Work out the finished part from the listing and answer in its coordinate system (mm). Face numbers are marked on the shaded views. A direction names the side the tool comes from. Coordinates: 2 decimals unless noted, no trailing zeros. Order: outer loops, then holes, each group sorted by start corner. A loop starts at its lowest first (then second) coordinate and runs counter-clockwise, first axis right, second up. Notation, with made-up numbers: M 60,23.25 L 75,23.25 A17 cw 75,35.25 Z; hole C -22.5,34 d4. An arc over 180 degrees is marked long. Answer in a Markdown table with one row per item. Add a question column.
Item 1: The part is cut by section A-A (x = 0). Write down the section's boundary in (y, z).
Item 2: Which of the six approach directions +Z, -Z, +X, -X, +Y, -Y give full straight-line access (tool end or side, diameter ignored) to the marked faces 1 and 2?
Item 3: The part is cut by section C-C (y = 11). Write down the section's boundary in (x, z), then the cut area to 3 significant figures.
Item 4: Flat-ended cylindrical pins translate along their axes: pin 1 Ø12 at (x, y) = (27.5, 4) entering from -Z; pin 2 Ø8 at (x, z) = (5.79, -4.21) entering from +Y; pin 3 Ø4 at (x, y) = (27, 4.5) entering from +Z; pin 4 Ø13.5 at (x, z) = (0, 0) entering from +Y. Find the tip coordinate at first contact, or state that the pin passes through.
Item 5: The part is cut by section B-B (z = 6.5). Write down the section's boundary in (x, y), then the cut area to 3 significant figures.
Item 6: Consider line 1 (X direction, y = 4.75, z = 8.5); line 2 (Y direction, x = -11, z = -0.5); line 3 (X direction, y = 3, z = -7.5). Determine where each line is inside the solid, lowest interval first. Write a range as from..to.
Item 7: The mould has two halves that part along Z. Classify the marked faces 3, 4, 5 and 6: released by +Z, released by -Z, zero draft, split by the parting line, or undercut.
Item 8: The part is cut by section D-D (x = 31.5). Write down the section's boundary in (y, z).
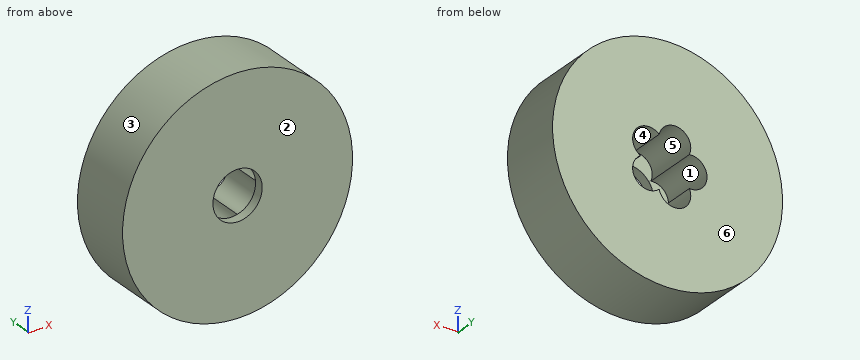
from build123d import *

# Parameters (mm, degrees)
SKETCH1_R           = 35
BOSS_EXTRUDE1_DEPTH = 20
SKETCH2_R           = 7.5
CUT_EXTRUDE1_DEPTH  = 54.38539126
SKETCH3_R           = 4.855176947
CUT_EXTRUDE2_DEPTH  = 17.075259
CIRPATTERN1_START   = 2.924741176
CIRPATTERN1_DEPTH   = 17.075258824


# Read off the part's stored shape, not the designer's step: CirPattern1
with BuildPart() as part:
    # Sketch1 → Boss-Extrude1 (new body)
    with BuildSketch(Plane(origin=(0, 0, 0), x_dir=(1, 0, 0), z_dir=(0, 1, 0))):
        with Locations(Location((0, 0, 0), (0, 0, 270))):
            Circle(SKETCH1_R)
    extrude(amount=BOSS_EXTRUDE1_DEPTH)

    # Sketch2 → Cut-Extrude1 (cut, through all)
    with BuildSketch(Plane(origin=(0, 0, 0), x_dir=(1, 0, 0), z_dir=(0, 1, 0))):
        with Locations(Location((0, 0, 0), (0, 0, 270))):
            Circle(SKETCH2_R)
    extrude(amount=CUT_EXTRUDE1_DEPTH, mode=Mode.SUBTRACT)

    # Sketch3 → Cut-Extrude2 (cut)
    with BuildSketch(Plane(origin=(0, 20, 0), x_dir=(1, 0, 0), z_dir=(0, 1, 0))):
        with Locations((-7.156774824, 0)):
            Circle(SKETCH3_R)
    extrude(amount=-CUT_EXTRUDE2_DEPTH, mode=Mode.SUBTRACT)

    # CirPattern1 outline → CirPattern1 (cut)
    with BuildSketch(Plane(origin=(0, 0, 0), x_dir=(1, 0, 0), z_dir=(0, 1, 0)).offset(CIRPATTERN1_START)):
        with BuildLine():
            ThreePointArc((-5.861347098, -4.679167682), (-6.250311255, -4.769807857), (-6.645409144, -4.828172359))
            ThreePointArc((-6.645409144, -4.828172359), (-3.711897233, -11.424045006), (2.538320424, -7.812146981))
            ThreePointArc((2.538320424, -7.812146981), (9.717873119, -7.060448103), (8.214177441, 0))
            ThreePointArc((8.214177441, 0), (9.717873119, 7.060448103), (2.538320424, 7.812146981))
            ThreePointArc((2.538320424, 7.812146981), (-3.711897233, 11.424045006), (-6.645409144, 4.828172359))
            ThreePointArc((-6.645409144, 4.828172359), (-6.250311255, 4.769807857), (-5.861347098, 4.679167682))
            ThreePointArc((-5.861347098, 4.679167682), (7.5, 0), (-5.861347098, -4.679167682))
        make_face()
    extrude(amount=CIRPATTERN1_DEPTH, mode=Mode.SUBTRACT)


solid = part.part
Reply:
| question | item | result |
|---|---|---|
| 1 | outline | M 0,-35 L 20,-35 L 20,-11.13 L 2.92,-11.13 L 2.92,-7.5 L 0,-7.5 Z; M 0,7.5 L 2.92,7.5 L 2.92,11.13 L 20,11.13 L 20,35 L 0,35 Z |
| 2 | face 1 | +Y |
| 2 | face 2 | +Z, -Z, +X, -X, -Y |
| 3 | outline | C 0,0 d70; hole M -6.65,-4.83 A4.86 ccw long 2.54,-7.81 A4.86 ccw long 8.21,0 A4.86 ccw long 2.54,7.81 A4.86 ccw long -6.65,4.83 A4.86 ccw long Z |
| 3 | area | 3,480 mm2 |
| 4 | pin 1 | stops at z = -27.62 |
| 4 | pin 2 | stops at y = 2.92 |
| 4 | pin 3 | stops at z = 24.49 |
| 4 | pin 4 | passes through |
| 5 | outline | M -34.39,0 L -3.74,0 L -3.74,2.92 L -7.06,2.92 L -7.06,20 L -34.39,20 Z; M 3.74,0 L 34.39,0 L 34.39,20 L 10.07,20 L 10.07,2.92 L 3.74,2.92 Z |
| 5 | area | 1,060 mm2 |
| 6 | line 1 | x = -33.95..-6.76, 2.34..3.52, 8.06..33.95 |
| 6 | line 2 | y = 0..2.92 |
| 6 | line 3 | x = -34.19..-7.02, 9.36..34.19 |
| 7 | face 3 | split by the parting line |
| 7 | face 4 | undercut |
| 7 | face 5 | undercut |
| 7 | face 6 | zero draft |
| 8 | outline | M 0,-15.26 L 20,-15.26 L 20,15.26 L 0,15.26 Z |
